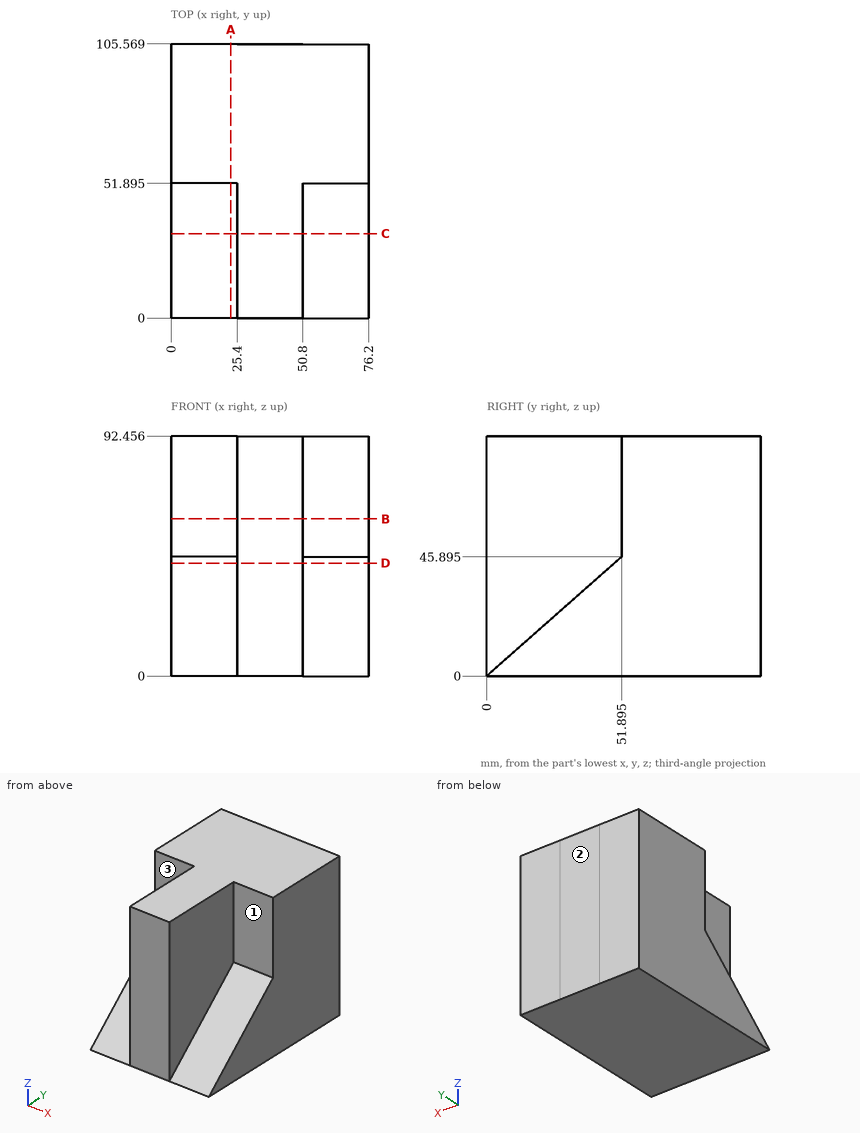
Verification items for this drawing (mm, ordinates from the low corner). A direction names the side the tool comes from. Round coordinates to 2 decimals unless told otherwise and drop trailing zeros. Order: outer loops, then holes, each group sorted by start corner. A loop starts at its lowest first (then second) coordinate and runs counter-clockwise, first axis right, second up. Notation, with made-up numbers: (21.5, 32) - (64.5, 32) arc R16 cw to (64.5, 59) - close; hole circle Ø6 at (-11.5, -22.75). An arc over 180 degrees is marked (long way). Use CSV: the item, a comma, the result in double quotes. Start each with the question number.
1) Section check D-D, the plane z = 43.5. Record the cut outline in (x, y), plus the area to 3 significant figures.
2) Section check A-A, the plane x = 23. Record the cut outline in (y, z) (1 decimal).
3) Section check C-C, the plane y = 32.5. Record the cut outline in (x, z).
4) Access from +Z, -Z, +X, -X, +Y, -Y to the whole of each face (thin tool, end or side, straight path). Record for the marked faces 1, 2 and 3.
5) Section check B-B, the plane z = 60.5. Record the cut outline in (x, y) (1 decimal), plus the area to 3 significant figures.
6) Go/stop test with flat-tipped pins: P1, Ø20.5, axis at x = 58, z = 68.5, coming from the -Y side; P2, Ø5, axis at x = 57, z = 37, coming from the -Y side; P3, Ø1, axis at x = 21.5, z = 16, coming from the -Y side (1 decimal); P4, Ø1, axis at y = 19.5, z = 22.5, coming from the +X side. Record where each tip stops, or that it passes through.
7) Thickness scan on L1, parallel to X at y = 48, z = 52; L2, parallel to Y at x = 5, z = 46.5 (1 decimal); L3, parallel to Y at x = 63, z = 12.5 (1 decimal). Record the ranges inside material, lowest first.
Answers:
1,outline,"(0, 49.19) - (25.4, 49.19) - (25.4, 0) - (50.8, 0) - (50.8, 49.19) - (76.2, 49.19) - (76.2, 105.57) - (0, 105.57) - close"
1,area,"5,550 mm²"
2,outline,"(0, 0) - (105.6, 0) - (105.6, 92.5) - (51.9, 92.5) - (51.9, 45.9) - close"
3,outline,"(0, 0) - (76.2, 0) - (76.2, 28.74) - (50.8, 28.74) - (50.8, 92.46) - (25.4, 92.46) - (25.4, 28.74) - (0, 28.74) - close"
4,face 1,"+Z, +X, -Y"
4,face 2,"+Z, -Z, +X, -X, +Y"
4,face 3,"+Z, -X, -Y"
5,outline,"(0, 51.9) - (25.4, 51.9) - (25.4, 0) - (50.8, 0) - (50.8, 51.9) - (76.2, 51.9) - (76.2, 105.6) - (0, 105.6) - close"
5,area,"5,410 mm²"
6,P1,"stops at y = 0"
6,P2,"stops at y = 39.01"
6,P3,"stops at y = 17.5"
6,P4,"stops at x = 50.8"
7,L1,"x = 25.4 to 50.8"
7,L2,"y = 51.9 to 105.6"
7,L3,"y = 14.1 to 105.6"
